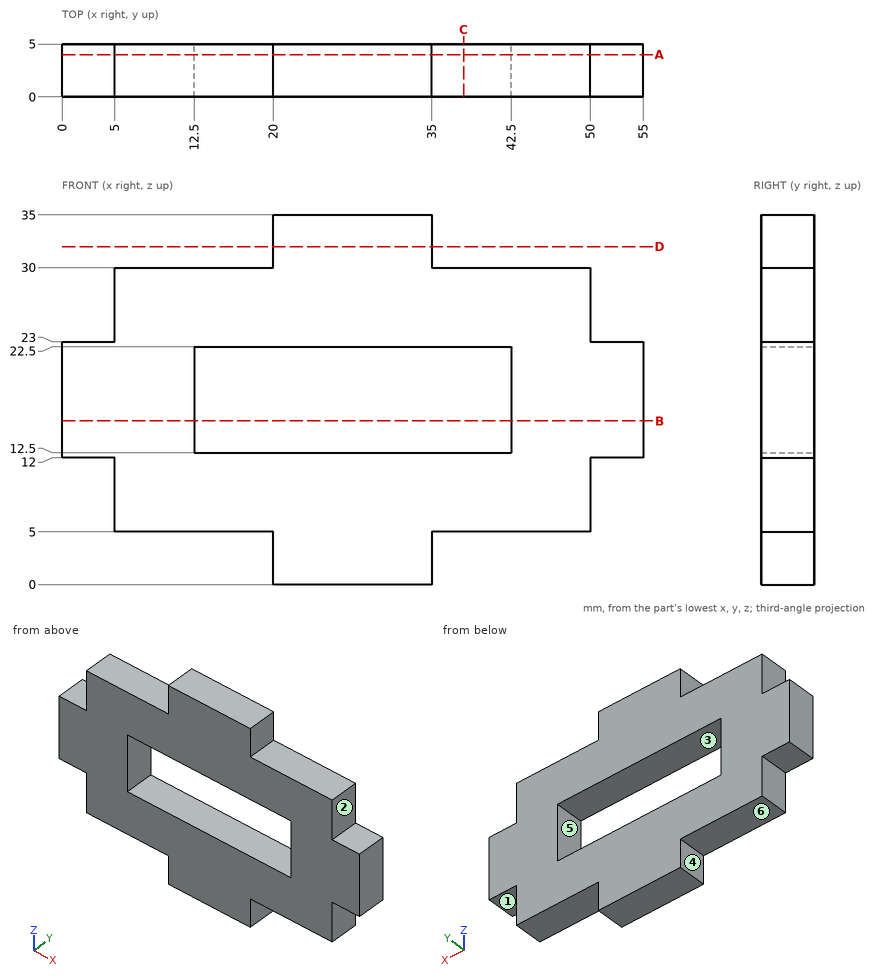
Could you check a few things on this drawing? It's one solid part, dimensions in mm from its lowest x, y, z. A direction names the side the tool comes from. Coordinates: 2 decimals unless noted, no trailing zeros. Order: outer loops, then holes, each group sorted by start corner. A loop starts at its lowest first (then second) coordinate and runs counter-clockwise, first axis right, second up. Notation, with made-up numbers: M -37,-27 L 0,-27 A30 cw 0,-3 Z; hole C 86,54.25 d7. An arc over 180 degrees is marked long. Answer as CSV lines item,"result".
(1) If we mould it in two halves opening along X, with no side actions, what happens to the marked faces 4, 5 and 6? For each: released by +X, released by -X, zero draft, split by the parting line, or undercut.
Geometry check:
face 4,"released by -X"
face 5,"undercut"
face 6,"zero draft"
(2) On a 3-axis mill with a long thin cutter (end or side, diameter ignored), from which of +Z, -Z, +X, -X, +Y, -Y can I reach the whole of each face in a straight line? I mean the marked faces 1, 2 and 3. Say none if no direction works.
Geometry check:
face 1,"-Z, +X, +Y, -Y"
face 2,"+Z, +X, +Y, -Y"
face 3,"+Y, -Y"
(3) Suppose I cut it at A-A on y = 4. Please give me the cut outline in (x, z).
Geometry check:
outline,"M 0,12 L 5,12 L 5,5 L 20,5 L 20,0 L 35,0 L 35,5 L 50,5 L 50,12 L 55,12 L 55,23 L 50,23 L 50,30 L 35,30 L 35,35 L 20,35 L 20,30 L 5,30 L 5,23 L 0,23 Z; hole M 12.5,12.5 L 42.5,12.5 L 42.5,22.5 L 12.5,22.5 Z"
(4) Suppose I cut it at D-D on z = 32. Please give me the cut outline in (x, y).
Geometry check:
outline,"M 20,0 L 35,0 L 35,5 L 20,5 Z"
(5) I'm going to push flat-ended pins straight in: pin 1 (2.5 mm diameter, centred on x = 52.5, y = 2.5, fed in from -Z); pin 2 (1.5 mm diameter, centred on y = 1.5, z = 32.5, fed in from -X); pin 3 (2.5 mm diameter, centred on x = 52, y = 1.5, fed in from +Z). Where does each tip first touch, or does it pass through?
Geometry check:
pin 1,"z = 12"
pin 2,"x = 20"
pin 3,"z = 23"
(6) Please list where these lines run through material, in increasing order: L1, parallel to Z at x = 28, y = 2.1; L2, parallel to X at y = 1.4, z = 14; L3, parallel to Z at x = 19, y = 4.1.
Geometry check:
L1,"0 to 12.5, 22.5 to 35"
L2,"0 to 12.5, 42.5 to 55"
L3,"5 to 12.5, 22.5 to 30"
(7) Suppose I cut it at C-C on x = 38. Please give me the cut outline in (y, z), plus the area to 3 significant figures.
Geometry check:
outline,"M 0,5 L 5,5 L 5,12.5 L 0,12.5 Z; M 0,22.5 L 5,22.5 L 5,30 L 0,30 Z"
area,"75.0 mm^2"
(8) Suppose I cut it at B-B on z = 15.5. Please give me the cut outline in (x, y).
Geometry check:
outline,"M 0,0 L 12.5,0 L 12.5,5 L 0,5 Z; M 42.5,0 L 55,0 L 55,5 L 42.5,5 Z"
